```python
from build123d import *

# Parameters (mm, degrees)
SKETCH1_W           = 151
SKETCH1_H           = 90
BOSS_EXTRUDE1_DEPTH = 3
SKETCH2_R           = 1.75
CUT_EXTRUDE1_DEPTH  = 176.812400018
FILLET1_R           = 2
SKETCH3_W           = 25.1
SKETCH3_H           = 3.1
CUT_EXTRUDE2_DEPTH  = 176.812400018


with BuildPart() as part:
    # Sketch1 → Boss-Extrude1 (new body)
    with BuildSketch(Plane(origin=(0, 0, 0), x_dir=(1, 0, 0), z_dir=(0, 1, 0))):
        with Locations((75.5, 45)):
            Rectangle(SKETCH1_W, SKETCH1_H)
    extrude(amount=BOSS_EXTRUDE1_DEPTH)

    # Sketch2 → Cut-Extrude1 (cut, through all)
    with BuildSketch(Plane(origin=(0, 3, 0), x_dir=(1, 0, 0), z_dir=(0, 1, 0))):
        with Locations(Location((146, 86, 0), (0, 0, 270))):
            Circle(SKETCH2_R)
        with Locations(Location((146, 4, 0), (0, 0, 270))):
            Circle(SKETCH2_R)
        with Locations(Location((6, 86, 0), (0, 0, 270))):
            Circle(SKETCH2_R)
        with Locations(Location((6, 4, 0), (0, 0, 270))):
            Circle(SKETCH2_R)
    extrude(amount=-CUT_EXTRUDE1_DEPTH, mode=Mode.SUBTRACT)

    # Fillet1
    fillet1_edges = [part.edges().sort_by_distance(p)[0] for p in [
        (0, 1.5, -90),
        (151, 1.5, -90),
        (151, 1.5, 0),
        (0, 1.5, 0),
    ]]
    fillet(fillet1_edges, radius=FILLET1_R)

    # Sketch3 → Cut-Extrude2 (cut, through all)
    with BuildSketch(Plane(origin=(0, 3, 0), x_dir=(1, 0, 0), z_dir=(0, 1, 0))):
        with Locations((97.55, 4.55)):
            Rectangle(SKETCH3_W, SKETCH3_H)
        with Locations((128.45, 4.55)):
            Rectangle(SKETCH3_W, SKETCH3_H)
    extrude(amount=-CUT_EXTRUDE2_DEPTH, mode=Mode.SUBTRACT)


solid = part.part
```
For this review, take the finished solid that the model builds, in its own axes (mm). A direction names the side the tool comes from. Round coordinates to 2 decimals unless told otherwise and drop trailing zeros. Write each loop counter-clockwise with the first axis right and the second up, starting at its lowest first coordinate (ties: lowest second). Pieces come first, ordered by that corner, then holes. Notation, with made-up numbers: (-18, 44) -> (-11, 44) arc R34 ccw to (-11, 82) -> close; hole circle Ø4 at (47.5, 15). An arc over 180 degrees is marked (long way). Use one line per item in the form item = value.
1) Clearance check with a flat-ended pin moving along its axis: pin 1 (10 mm diameter, centred on x = 19.5, z = -57.5, fed in from -Y). State where the tip first meets the part, or that it passes through.
Found:
pin_1 = 0
2) Take a section at B-B, the plane z = -86. Write out the cut boundary in (x, y), and give its area (3 significant figures).
Found:
outline = (0, 0) -> (4.25, 0) -> (4.25, 3) -> (0, 3) -> close; (7.75, 0) -> (144.25, 0) -> (144.25, 3) -> (7.75, 3) -> close; (147.75, 0) -> (151, 0) -> (151, 3) -> (147.75, 3) -> close
area = 432 mm2
3) To check wall thickness, follow L1, parallel to X at y = 1.2, z = -86; L2, parallel to X at y = 0.85, z = -4; L3, parallel to Z at x = 146, y = 1.3. State the ranges of each line that lie inside material, in increasing order. Write a range as from..to.
Found:
L1 = 0..4.25, 7.75..144.25, 147.75..151
L2 = 0..4.25, 7.75..85, 110.1..115.9, 141..144.25, 147.75..151
L3 = -90..-87.75, -84.25..-5.75, -2.25..0
4) Tool access review of faces 1 (the flat face through (74, 1, -90)), 2 (the flat face through (85, 2, -5)): name each direction out of +Z, -Z, +X, -X, +Y, -Y from which nothing blocks a thin tool from reaching the whole face with its end or side.
Found:
face_1 = -Z, +X, -X, +Y, -Y
face_2 = +Y, -Y
5) Take a section at A-A, the plane x = 146. Write out the cut boundary in (y, z), and give its area (3 significant figures).
Found:
outline = (0, -90) -> (3, -90) -> (3, -87.75) -> (0, -87.75) -> close; (0, -84.25) -> (3, -84.25) -> (3, -5.75) -> (0, -5.75) -> close; (0, -2.25) -> (3, -2.25) -> (3, 0) -> (0, 0) -> close
area = 249 mm2
6) Mouldability with a two-part tool opening along Z and no side actions: class faces 3 (the flat face through (74, 1, 0)), 4 (the flat face through (128, 2, -6.1)), 5 (the cylindrical face through (4.94, 1.52, -5.39)), 6 (the flat face through (74, 3, -46)) as +Z half, -Z half, draft (parallel to the pull), parting line (faces both ways), or undercut.
Found:
face_3 = +Z half
face_4 = undercut
face_5 = undercut
face_6 = draft
